Verification items for this drawing (mm, ordinates from the low corner). A direction names the side the tool comes from. Coordinates: 2 decimals unless noted, no trailing zeros. Loops run counter-clockwise (first coordinate to the right, second up) from the corner with the lowest first, then second, coordinate; pieces in that order, holes last. Notation, with made-up numbers: M 85,16.5 L 97,16.5 A26 cw 97,34.5 Z; hole C -18,37.25 d2. An arc over 180 degrees is marked long. Return JSON: item names as keys, results as strings.
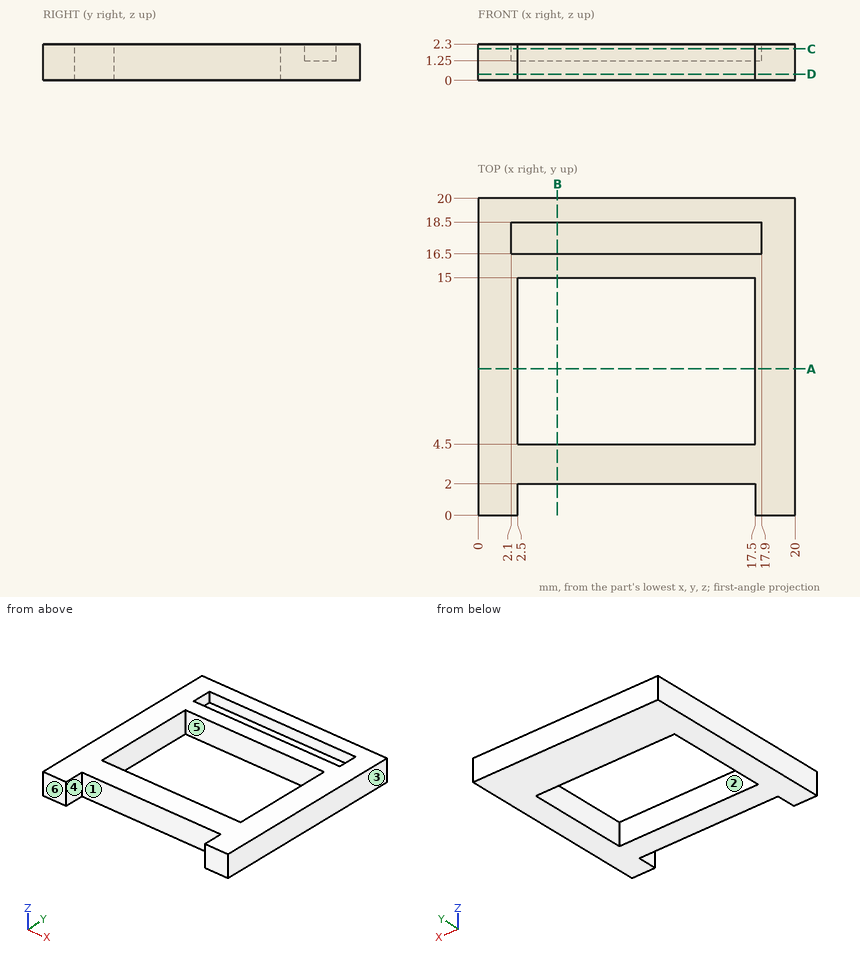
1) Go/stop test with a flat-tipped pin: pin 1 Ø1.2 at (x, z) = (10, 1) entering from -Y. Record where the tip stops, or that it passes through.
Answers:
{"pin 1": "y = 2"}
2) Section check B-B on x = 5. Record the cut outline in (y, z), then the cut area to 4 significant figures.
Answers:
{"outline": "M 2,0 L 4.5,0 L 4.5,2.3 L 2,2.3 Z; M 15,0 L 20,0 L 20,2.3 L 18.5,2.3 L 18.5,1.25 L 16.5,1.25 L 16.5,2.3 L 15,2.3 Z", "area": "15.15 mm²"}
3) Section check A-A on y = 9.25. Record the cut outline in (x, z), then the cut area to 3 significant figures.
Answers:
{"outline": "M 0,0 L 2.5,0 L 2.5,2.3 L 0,2.3 Z; M 17.5,0 L 20,0 L 20,2.3 L 17.5,2.3 Z", "area": "11.5 mm²"}
4) Section check D-D on z = 0.4. Record the cut outline in (x, y), then the cut area to 4 significant figures.
Answers:
{"outline": "M 0,0 L 2.5,0 L 2.5,2 L 17.5,2 L 17.5,0 L 20,0 L 20,20 L 0,20 Z; hole M 2.5,4.5 L 17.5,4.5 L 17.5,15 L 2.5,15 Z", "area": "212.5 mm²"}
5) Draft check along Y on the marked faces 1, 2 and 3. Enter one of: +Y half, -Y half, draft (parallel to the pull), parting line (faces both ways), or undercut.
Answers:
{"face 1": "-Y half", "face 2": "undercut", "face 3": "draft"}
6) Section check C-C on z = 2. Record the cut outline in (x, y).
Answers:
{"outline": "M 0,0 L 2.5,0 L 2.5,2 L 17.5,2 L 17.5,0 L 20,0 L 20,20 L 0,20 Z; hole M 2.1,16.5 L 17.9,16.5 L 17.9,18.5 L 2.1,18.5 Z; hole M 2.5,4.5 L 17.5,4.5 L 17.5,15 L 2.5,15 Z"}
7) Scan lines: line 1 along Y through (x, z) = (11.25, 1.45); line 2 along Y through (x, z) = (13.75, 0.95); line 3 along X through (y, z) = (6.75, 1.4). Record each from-to range of solid material in increasing order. Write a range as [from, to].
Answers:
{"line 1": "[2, 4.5], [15, 16.5], [18.5, 20]", "line 2": "[2, 4.5], [15, 20]", "line 3": "[0, 2.5], [17.5, 20]"}
8) Set-up check for the marked faces 4, 5 and 6: record each of +Z, -Z, +X, -X, +Y, -Y from which the full face is reachable in a straight line by a thin tool's end or side.
Answers:
{"face 4": "+Z, -Z, -Y", "face 5": "+Z, -Z", "face 6": "+Z, -Z, +X, -X, -Y"}
